```python
from build123d import *

# Parameters (mm, degrees)
SKETCH1_R           = 20
BOSS_EXTRUDE1_DEPTH = 30
SKETCH2_R           = 5
BOSS_EXTRUDE2_DEPTH = 5
CUT_EXTRUDE1_REACH  = 47
CUT_EXTRUDE2_START  = -25
SKETCH4_R           = 15
SKETCH4_R_2         = 5
CUT_EXTRUDE2_DEPTH  = 25
SKETCH5_R           = 15
CUT_EXTRUDE3_DEPTH  = 2


with BuildPart() as part:
    # Sketch1 → Boss-Extrude1 (new body)
    with BuildSketch(Plane(origin=(0, 0, 0), x_dir=(0, 0, -1), z_dir=(1, 0, 0))):
        Circle(SKETCH1_R)
    extrude(amount=BOSS_EXTRUDE1_DEPTH)

    # Sketch2 → Boss-Extrude2 (add)
    with BuildSketch(Plane.ZY):
        with Locations(Location((0, 0, 0), (0, 0, 180))):
            Circle(SKETCH2_R)
    extrude(amount=BOSS_EXTRUDE2_DEPTH)

    # Sketch3 → Cut-Extrude1 (cut, up to next)
    with BuildSketch(Plane(origin=(30, 0, 0), x_dir=(0, 0, -1), z_dir=(1, 0, 0)), mode=Mode.PRIVATE) as cut_extrude1_sk1:
        with BuildLine():
            Line((0, 5), (0, 15))
            ThreePointArc((0, 15), (-2.018355219, 14.863587797), (-4, 14.456832295))
            Line((-4, 14.456832295), (-2, 4.582575695))
            ThreePointArc((-2, 4.582575695), (-1.021548218, 4.894531565), (0, 5))
        make_face()
    cut_extrude1_tool1 = extrude(cut_extrude1_sk1.sketch, amount=-CUT_EXTRUDE1_REACH, mode=Mode.PRIVATE) & part.part
    # Sketch3 → Cut-Extrude1 (cut, up to next)
    with BuildSketch(Plane(origin=(30, 0, 0), x_dir=(0, 0, -1), z_dir=(1, 0, 0)), mode=Mode.PRIVATE) as cut_extrude1_sk2:
        with BuildLine():
            ThreePointArc((4, 14.456832295), (2.018355219, 14.863587797), (0, 15))
            Line((0, 15), (0, 5))
            ThreePointArc((0, 5), (1.021548218, 4.894531565), (2, 4.582575695))
            Line((2, 4.582575695), (4, 14.456832295))
        make_face()
    cut_extrude1_tool2 = extrude(cut_extrude1_sk2.sketch, amount=-CUT_EXTRUDE1_REACH, mode=Mode.PRIVATE) & part.part
    # Sketch3 → Cut-Extrude1 (cut, up to next)
    with BuildSketch(Plane(origin=(30, 0, 0), x_dir=(0, 0, -1), z_dir=(1, 0, 0)), mode=Mode.PRIVATE) as cut_extrude1_sk3:
        with BuildLine():
            Line((-3.740254487, 3.3182068), (-12.513196581, 8.271632929))
            ThreePointArc((-12.513196581, 8.271632929), (-14.265847744, 4.635254916), (-14.985332536, 0.663180799))
            Line((-14.985332536, 0.663180799), (-4.976322465, -0.486019265))
            ThreePointArc((-4.976322465, -0.486019265), (-4.755282581, 1.545084972), (-3.740254487, 3.3182068))
        make_face()
    cut_extrude1_tool3 = extrude(cut_extrude1_sk3.sketch, amount=-CUT_EXTRUDE1_REACH, mode=Mode.PRIVATE) & part.part
    # Sketch3 → Cut-Extrude1 (cut, up to next)
    with BuildSketch(Plane(origin=(30, 0, 0), x_dir=(0, 0, -1), z_dir=(1, 0, 0)), mode=Mode.PRIVATE) as cut_extrude1_sk4:
        with BuildLine():
            Line((-5.26144484, -14.04696402), (-1.075536422, -4.88295212))
            ThreePointArc((-1.075536422, -4.88295212), (-2.938926261, -4.045084972), (-4.3116044, -2.531811111))
            Line((-4.3116044, -2.531811111), (-11.733580795, -9.344682002))
            ThreePointArc((-11.733580795, -9.344682002), (-8.816778784, -12.135254916), (-5.26144484, -14.04696402))
        make_face()
    cut_extrude1_tool4 = extrude(cut_extrude1_sk4.sketch, amount=-CUT_EXTRUDE1_REACH, mode=Mode.PRIVATE) & part.part
    # Sketch3 → Cut-Extrude1 (cut, up to next)
    with BuildSketch(Plane(origin=(30, 0, 0), x_dir=(0, 0, -1), z_dir=(1, 0, 0)), mode=Mode.PRIVATE) as cut_extrude1_sk5:
        with BuildLine():
            ThreePointArc((4.3116044, -2.531811111), (2.938926261, -4.045084972), (1.075536422, -4.88295212))
            Line((1.075536422, -4.88295212), (5.26144484, -14.04696402))
            ThreePointArc((5.26144484, -14.04696402), (8.816778784, -12.135254916), (11.733580795, -9.344682002))
            Line((11.733580795, -9.344682002), (4.3116044, -2.531811111))
        make_face()
    cut_extrude1_tool5 = extrude(cut_extrude1_sk5.sketch, amount=-CUT_EXTRUDE1_REACH, mode=Mode.PRIVATE) & part.part
    # Sketch3 → Cut-Extrude1 (cut, up to next)
    with BuildSketch(Plane(origin=(30, 0, 0), x_dir=(0, 0, -1), z_dir=(1, 0, 0)), mode=Mode.PRIVATE) as cut_extrude1_sk6:
        with BuildLine():
            ThreePointArc((14.985332536, 0.663180799), (14.265847744, 4.635254916), (12.513196581, 8.271632929))
            Line((12.513196581, 8.271632929), (3.740254487, 3.3182068))
            ThreePointArc((3.740254487, 3.3182068), (4.67446641, 1.774644692), (5, 0))
            ThreePointArc((5, 0), (4.994077108, -0.243297838), (4.976322465, -0.486019265))
            Line((4.976322465, -0.486019265), (14.985332536, 0.663180799))
        make_face()
    cut_extrude1_tool6 = extrude(cut_extrude1_sk6.sketch, amount=-CUT_EXTRUDE1_REACH, mode=Mode.PRIVATE) & part.part
    add(cut_extrude1_tool1.solids().sort_by_distance((30, 10.385553, 1.567824))[0], mode=Mode.SUBTRACT)
    add(cut_extrude1_tool2.solids().sort_by_distance((30, 10.385553, -1.567824))[0], mode=Mode.SUBTRACT)
    add(cut_extrude1_tool3.solids().sort_by_distance((30, 3.209313, 9.877248))[0], mode=Mode.SUBTRACT)
    add(cut_extrude1_tool4.solids().sort_by_distance((30, -8.402089, 6.104475))[0], mode=Mode.SUBTRACT)
    add(cut_extrude1_tool5.solids().sort_by_distance((30, -8.402089, -6.104475))[0], mode=Mode.SUBTRACT)
    add(cut_extrude1_tool6.solids().sort_by_distance((30, 3.209313, -9.877248))[0], mode=Mode.SUBTRACT)

    # Sketch4 → Cut-Extrude2 (cut)
    with BuildSketch(Plane.ZY.offset(CUT_EXTRUDE2_START)):
        with Locations(Location((0, 0, 0), (0, 0, 180))):
            Circle(SKETCH4_R)
        with Locations(Location((0, 0, 0), (0, 0, 185.578178478))):
            Circle(SKETCH4_R_2, mode=Mode.SUBTRACT)
    extrude(amount=CUT_EXTRUDE2_DEPTH, mode=Mode.SUBTRACT)

    # Sketch5 → Cut-Extrude3 (cut)
    with BuildSketch(Plane(origin=(30, 0, 0), x_dir=(0, 0, -1), z_dir=(1, 0, 0))):
        Circle(SKETCH5_R)
    extrude(amount=-CUT_EXTRUDE3_DEPTH, mode=Mode.SUBTRACT)


solid = part.part
```
Here's how the part is built. I have some questions about the finished solid (model axes, mm). A direction names the side the tool comes from. Give positions to 0.01 mm unless a question says otherwise; leave off trailing zeros. Loops run counter-clockwise (first coordinate to the right, second up) from the corner with the lowest first, then second, coordinate; pieces in that order, holes last. Notation, with made-up numbers: M -33.5,42.5 L 21.5,42.5 A22 cw 21.5,80.5 Z; hole C -22.5,0.5 d5. An arc over 180 degrees is marked long. Use one line per item in the form item = value. Start each with the question number.
Q1. Will these pins go through, and if not, where does the flat tip stop? pin 1 Ø4 at (y, z) = (-9, 13.5) entering from -X; pin 2 Ø14.5 at (y, z) = (0.5, -5.5) entering from +X; pin 3 Ø5 at (x, y) = (21.5, 11.5) entering from -Z.
Q2. Thinking about a two-plate mould opening in Z: for faces 1 (the flat face through (26.52, -5.89, 7.97)), 2 (the flat face through (0, 15, -3)), 3 (the cylindrical face through (14.79, -19.524, 4.336)), which applies, +Z half, -Z half, draft (parallel to the pull), parting line (faces both ways), or undercut?
Q3. If we section it at D-D (z = -11): Write out the boundary of the cut face in (x, y).
Q4. If we section it at B-B (x = 26): Write out the boundary of the cut face in (y, z), then the cut area to 3 significant figures.
Q5. If we section it at C-C (z = 14): Write out the boundary of the cut face in (x, y), then the cut area to 3 significant figures.
Q6. If we section it at A-A (x = 9): Write out the boundary of the cut face in (y, z).
Q7. I need wall thicknesses on line 1 along Y through (x, z) = (15, -1.5); line 2 along Z through (x, y) = (23.5, -4); line 3 along Y through (x, z) = (12.5, 3). Which ranges of each line are inside material? Lowest first, please.
Q8. Which directions (+Z, -Z, +X, -X, +Y, -Y) give clear straight access to the entire face, cutting with the end or side of a thin tool? Please do faces 4 (the flat face through (-5, 0, 0)), 5 (the flat face through (25, -3, -11)), 6 (the flat face through (26.52, 5.83, -8.19)), 7 (the flat face through (30, 15, -3)), 8 (the flat face through (28, 0, 0)).
Taken from the geometry:
q1.pin_1 = 0
q1.pin_2 = 28
q1.pin_3 = -17.86
q2.face_1 = undercut
q2.face_2 = draft
q2.face_3 = parting line
q3.outline = M 0,-16.7 L 30,-16.7 L 30,-10.2 L 0,-10.2 Z; M 0,10.2 L 25,10.2 L 25,7.42 L 28,7.42 L 28,10.2 L 30,10.2 L 30,16.7 L 0,16.7 Z; M 25,-8.67 L 28,-8.67 L 28,0.21 L 25,0.21 Z
q4.outline = C 0,0 d40; hole M -14.05,-5.26 A15 ccw -9.34,-11.73 L -2.53,-4.31 A5 cw -4.88,-1.08 Z; hole M -14.05,5.26 L -4.88,1.08 A5 cw -2.53,4.31 L -9.34,11.73 A15 ccw Z; hole M -0.49,-4.98 L 0.66,-14.99 A15 ccw 8.27,-12.51 L 3.32,-3.74 A5 cw Z; hole M -0.49,4.98 A5 cw 3.32,3.74 L 8.27,12.51 A15 ccw 0.66,14.99 Z; hole M 4.58,-2 L 14.46,-4 A15 ccw 14.46,4 L 4.58,2 A5 cw Z
q4.area = 951 mm^2
q5.outline = M 0,-14.28 L 30,-14.28 L 30,-5.39 L 28,-5.39 L 28,0.55 L 25,0.55 L 25,-5.39 L 0,-5.39 Z; M 0,5.39 L 30,5.39 L 30,14.28 L 0,14.28 Z
q5.area = 552 mm^2
q6.outline = C 0,0 d40; C 0,0 d10; hole C 0,0 d30
q7.line_1 = -19.94 to -14.92, -4.77 to 4.77, 14.92 to 19.94
q7.line_2 = -19.6 to -14.46, -3 to 3, 14.46 to 19.6
q7.line_3 = -19.77 to -14.7, -4 to 4, 14.7 to 19.77
q8.face_4 = +Z, -Z, -X, +Y, -Y
q8.face_5 = -X
q8.face_6 = +X, -X
q8.face_7 = +Z, -Z, +X, +Y, -Y
q8.face_8 = +X
